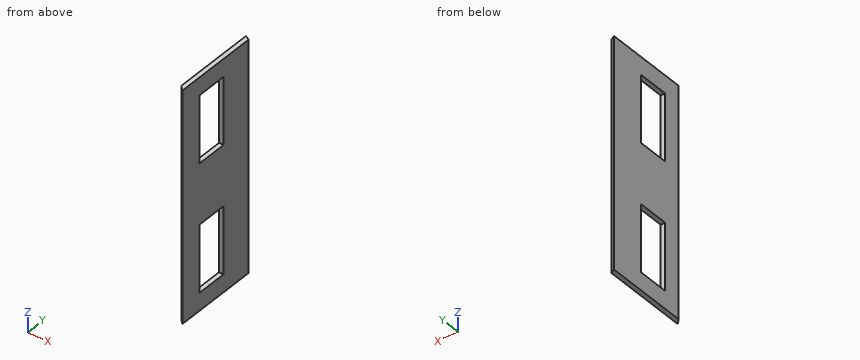
Autodesk Inventor part; units mm, degrees
ref_plane "YZ Plane" through (0, 0, 0) normal (1, 0, 0) x (0, 1, 0)
ref_plane "XZ Plane" through (0, 0, 0) normal (0, 1, 0) x (-1, 0, 0)
ref_plane "XY Plane" through (0, 0, 0) normal (0, 0, 1) x (1, 0, 0)
sketch "Szkic1" plane through (0, 0, 0) normal (1, 0, 0) x (0, 1, 0)
  line L0 (9.1767, 36.8868) -> (23.0303, 36.8868)
  line L1 (23.0303, 36.8868) -> (23.0303, 8.0794)
  line L2 (22.5303, 5.7086) -> (9.1767, 5.7086)
  line L3 (9.1767, 5.7086) -> (9.1767, 36.8868)
  line L4 (0, 100) -> (39.1311, 100)
  line L5 (39.1311, 0) -> (0, 0)
  line L6 (23.0303, 63.1132) -> (9.1767, 63.1132)
  line L7 (9.1767, 63.1132) -> (9.1767, 94.2914)
  line L8 (9.1767, 94.2914) -> (23.0303, 94.2914)
  line L9 (23.0303, 94.2914) -> (23.0303, 63.1132)
  line L10 (39.1311, 100) -> (40.1311, 100)
  line L11 (40.1311, 0) -> (39.1311, 0)
  line L12 (40.1311, 100) -> (40.1311, 0)
  line L13 (-0.559, 100) -> (-0.1118, 100)
  line L14 (-0.559, 100) -> (-0.559, 0)
  line L15 (-0.1118, 0) -> (-0.559, 0)
  line L16 (-0.1118, 100) -> (0.1125, 100)
  line L17 (23.0303, 8.0794) -> (23.0303, 5.7086)
  line L18 (23.0303, 5.7086) -> (22.5303, 5.7086)
  line L19 (40.1311, 100) -> (-0.559, 100)
  line L20 (-0.559, 100) -> (-0.559, 0)
  line L21 (-0.559, 0) -> (40.1311, 0)
  line L22 (40.1311, 0) -> (40.1311, 100)
  point P0 (11.7487, 100)
extrude "Wyciągnięcie proste1" add sketch "Szkic1" along normal blind 2
chamfer "Faza1" distance 2 angle 45 2 edges at (0, -0.559, 50) (2, 40.1311, 50)
sketch "Szkic2" plane through (0, 1.441, 100) normal (0, 0, 1) x (1, 0, 0)
  line L0 (0, 37.0479) -> (-58.736, 68.461)
  line L1 (0, 37.0479) -> (5, 34.3738)
  line L2 (5, 34.3738) -> (2.5, 39)
  line L3 (2.5, 39) -> (-2, 40)
  line L4 (-2, 40) -> (-2.3739, 38.3175)
  point P0 (0, -1.441)
extrude "Wyciągnięcie proste2" cut sketch "Szkic2" against normal through all
sketch "Szkic3" plane through (2, 0, 0) normal (1, 0, 0) x (0, 0, -1)
  line L0 (-94.2914, 9.1767) -> (-94.2914, 23.0303)
  line L1 (-94.2914, 23.0303) -> (-63.1132, 23.0303)
  line L2 (-63.1132, 9.1767) -> (-94.2914, 9.1767)
  line L3 (-5.7086, 9.1767) -> (-36.8868, 9.1767)
  line L4 (-36.8868, 23.0303) -> (-5.7086, 23.0303)
  line L5 (-5.7086, 23.0303) -> (-5.7086, 9.1767)
  line L6 (-63.1132, 9.1767) -> (-94.2914, 9.1767)
  line L7 (-94.2914, 23.0303) -> (-92.2914, 23.0303)
  line L8 (-92.2914, 23.0303) -> (-92.2914, 9.1767)
  line L9 (-92.2914, 9.1767) -> (-94.2914, 9.1767)
  line L10 (-94.2914, 9.1767) -> (-94.2914, 23.0303)
  line L11 (-5.7086, 9.1767) -> (-36.8868, 9.1767)
  line L12 (-36.8868, 23.0303) -> (-5.7086, 23.0303)
  line L13 (-5.7086, 9.1767) -> (-7.7086, 9.1767)
  line L14 (-7.7086, 9.1767) -> (-7.7086, 23.0303)
  line L15 (-7.7086, 23.0303) -> (-5.7086, 23.0303)
  line L16 (-5.7086, 23.0303) -> (-5.7086, 9.1767)
  point P0 (0, 0)
  dimension "d7" = 2
  dimension "d8" = 2
extrude "Wyciągnięcie proste3" add sketch "Szkic3" against normal blind 2
properties part number "plug_nowy" material "Aluminium 6061"
Input: part model. Units: mm. Frame: model coordinates. Give positions to 0.01 mm unless a question says otherwise; leave off trailing zeros. Write each loop counter-clockwise with the first axis right and the second up, starting at its lowest first coordinate (ties: lowest second). Pieces come first, ordered by that corner, then holes.
Q1. Section C-C, the plane x = 1.3. Output: boundary loops of the cut face in (y, z), plus the area to 3 significant figures.
Q2. Material intervals for probe 1 along Z at (x, y) = (0.4, 22); probe 2 along Y at (x, z) = (0.95, 68); probe 3 along Y at (x, z) = (1.35, 66.5), sorted ascending.
Q3. Section B-B, the plane y = 16. Output: boundary loops of the cut face in (x, z), plus the area to 3 significant figures.
Q4. First-contact query: P1, Ø0.6, axis at x = 0.5, z = 82, coming from the +Y side; P2, Ø1, axis at x = 0.5, z = 23, coming from the -Y side. Flat tips, straight axial feed; report the tip coordinate or a pass-through.
Filled in:
1. outline: (0.14, 0) - (37.79, 0) - (37.79, 100) - (0.14, 100) - close; hole (9.18, 7.71) - (23.03, 7.71) - (23.03, 36.89) - (9.18, 36.89) - close; hole (9.18, 63.11) - (23.03, 63.11) - (23.03, 92.29) - (9.18, 92.29) - close
1. area: 2,960 mm2
2. probe 1: z = 0 to 7.71, 36.89 to 63.11, 92.29 to 100
2. probe 2: y = 0.49 to 9.18, 23.03 to 37.98
2. probe 3: y = 0.09 to 9.18, 23.03 to 37.77
3. outline: (0, 0) - (2, 0) - (2, 7.71) - (0, 7.71) - close; (0, 36.89) - (2, 36.89) - (2, 63.11) - (0, 63.11) - close; (0, 92.29) - (2, 92.29) - (2, 100) - (0, 100) - close
3. area: 83.3 mm2
4. P1: stops at y = 38.38
4. P2: stops at y = 0.44
